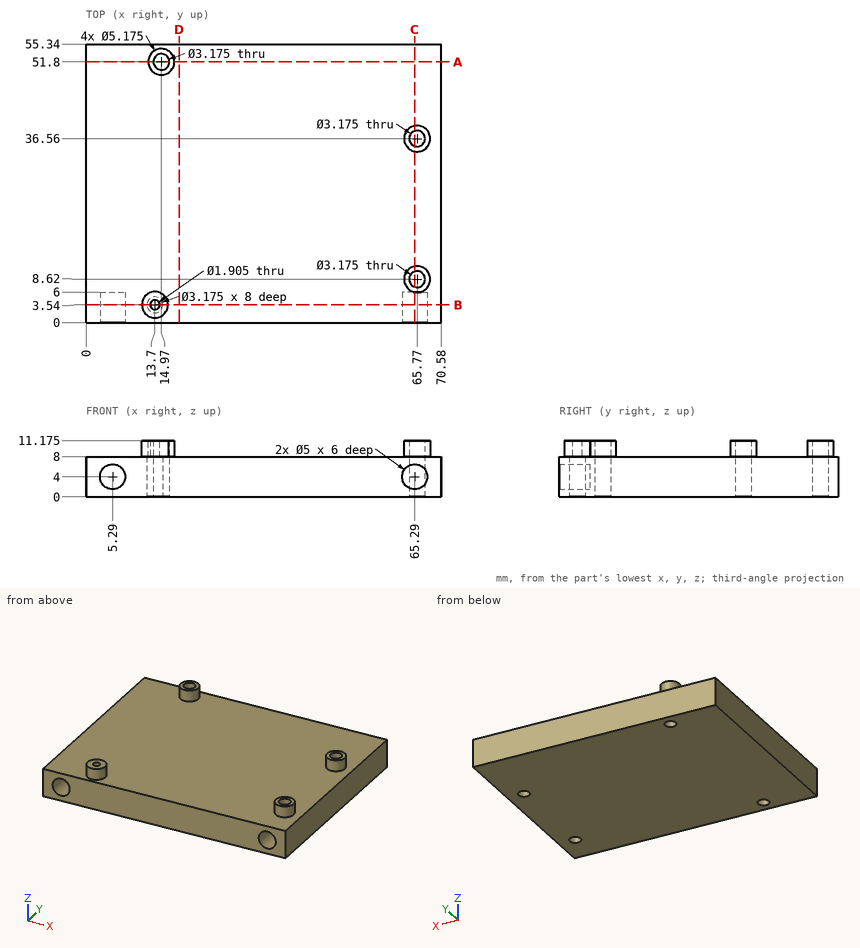
Study the drawing (mm; zero at the part's minimum x, y, z) and answer. Coordinates: 2 decimals unless noted, no trailing zeros. Write each loop counter-clockwise with the first axis right and the second up, starting at its lowest first coordinate (ties: lowest second). Pieces come first, ordered by that corner, then holes. Notation, with made-up numbers: (-12.75, -38.5) - (24.25, -38.5) arc R27 ccw to (24.25, -17.5) - close; hole circle Ø6 at (49.25, -18). An arc over 180 degrees is marked (long way). Answer as a JSON object with one key per item and string values.
Q1. Consider L1, parallel to Y at x = 65.77, z = 4.25; L2, parallel to Y at x = 14.5, z = 7.5; L3, parallel to Z at x = 65.29, y = 4.75. Determine where each line is inside the solid, lowest interval first. Write a range as from..to.
Results list:
{"L1": "y = 6..7.03, 10.21..34.97, 38.15..55.34", "L2": "y = 0..2.17, 4.91..50.28, 53.32..55.34", "L3": "z = 0..1.5, 6.5..8"}
Q2. Find section C-C (x = 65.29). Write down the section's boundary in (y, z) (3 decimals), plus the area to 3 significant figures.
Results list:
{"outline": "(0, 0) - (7.107, 0) - (7.107, 11.175) - (6.077, 11.175) - (6.077, 8) - (0, 8) - (0, 6.5) - (6, 6.5) - (6, 1.5) - (0, 1.5) - close; (10.133, 0) - (35.047, 0) - (35.047, 11.175) - (34.017, 11.175) - (34.017, 8) - (11.163, 8) - (11.163, 11.175) - (10.133, 11.175) - close; (38.073, 0) - (55.34, 0) - (55.34, 8) - (39.103, 8) - (39.103, 11.175) - (38.073, 11.175) - close", "area": "377 mm^2"}
Q3. Find section B-B (y = 3.54). Write down the section's boundary in (x, z) (1 decimal).
Results list:
{"outline": "(0, 0) - (12.1, 0) - (12.1, 8) - (12.7, 8) - (12.7, 11.2) - (11.1, 11.2) - (11.1, 8) - (0, 8) - close; (14.7, 8) - (15.3, 8) - (15.3, 0) - (70.6, 0) - (70.6, 8) - (16.3, 8) - (16.3, 11.2) - (14.7, 11.2) - close; hole circle Ø5 at (5.3, 4); hole circle Ø5 at (65.3, 4)"}
Q4. Find section A-A (y = 51.8). Write down the section's boundary in (x, z) (1 decimal).
Results list:
{"outline": "(0, 0) - (13.4, 0) - (13.4, 11.2) - (12.4, 11.2) - (12.4, 8) - (0, 8) - close; (16.6, 0) - (70.6, 0) - (70.6, 8) - (17.6, 8) - (17.6, 11.2) - (16.6, 11.2) - close"}
Q5. Find section D-D (x = 18.5). Write down the section's boundary in (y, z), plus the area to 3 significant figures.
Results list:
{"outline": "(0, 0) - (55.34, 0) - (55.34, 8) - (0, 8) - close", "area": "443 mm^2"}
Q6. Given pin 1 Ø3 at (x, y) = (65.77, 36.56) entering from -Z; pin 2 Ø10 at (x, y) = (57.5, 38) entering from +Z, each flat-ended and moving along its own axis, determine where each tip first touches the part or whether it passes through.
Results list:
{"pin 1": "passes through", "pin 2": "stops at z = 8"}
